Verification items for the finished model (mm, model axes). Face numbers are marked on the shaded views. A direction names the side the tool comes from. Round coordinates to 2 decimals unless told otherwise and drop trailing zeros. Write each loop counter-clockwise with the first axis right and the second up, starting at its lowest first coordinate (ties: lowest second). Pieces come first, ordered by that corner, then holes.
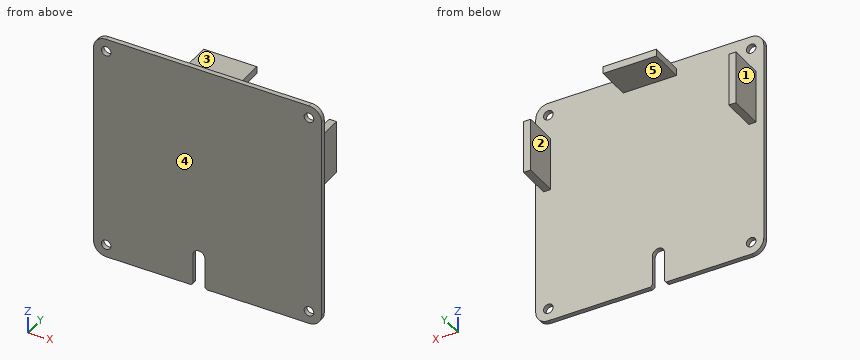
from build123d import *

# Parameters (mm, degrees)
BASE_PLATE_R            = 1.6
PCB_DEPTH               = 1.55
FILLET_1_R              = 1
SKETCH_2_W              = 2.4
SKETCH_2_H              = 17.8
SKETCH_2_W_2            = 17.8
SKETCH_2_H_2            = 2.4
LIDAR_PINS_DEPTH        = 8.5
SKETCH_3_W              = 2.4
SKETCH_3_H              = 17.8
SKETCH_3_W_2            = 17.8
SKETCH_3_H_2            = 2.4
LIDAR_PIN_HEADERS_DEPTH = 3


with BuildPart() as part:
    # Base plate → PCB (new body)
    with BuildSketch(Plane(origin=(0, 0, 0), x_dir=(1, 0, 0), z_dir=(0, 1, 0))):
        with BuildLine():
            ThreePointArc((-38.1, -33.9), (-36.869848481, -36.869848481), (-33.9, -38.1))
            Line((-33.9, -38.1), (33.9, -38.1))
            ThreePointArc((33.9, -38.1), (36.869848481, -36.869848481), (38.1, -33.9))
            Line((38.1, -33.9), (38.1, 33.9))
            ThreePointArc((38.1, 33.9), (36.869848481, 36.869848481), (33.9, 38.1))
            Line((33.9, 38.1), (-0.9, 38.1))
            Line((-0.9, 38.1), (-0.9, 27.4))
            ThreePointArc((-0.9, 27.4), (-2.9, 25.4), (-4.9, 27.4))
            Line((-4.9, 27.4), (-4.9, 38.1))
            Line((-4.9, 38.1), (-33.9, 38.1))
            ThreePointArc((-33.9, 38.1), (-36.869848481, 36.869848481), (-38.1, 33.9))
            Line((-38.1, 33.9), (-38.1, -33.9))
        make_face()
        with Locations(Location((-33.9, -33.9, 0), (0, 0, 90))):
            Circle(BASE_PLATE_R, mode=Mode.SUBTRACT)
        with Locations(Location((33.9, -33.9, 0), (0, 0, 90))):
            Circle(BASE_PLATE_R, mode=Mode.SUBTRACT)
        with Locations(Location((-33.9, 33.9, 0), (0, 0, 90))):
            Circle(BASE_PLATE_R, mode=Mode.SUBTRACT)
        with Locations(Location((33.9, 33.9, 0), (0, 0, 90))):
            Circle(BASE_PLATE_R, mode=Mode.SUBTRACT)
    extrude(amount=PCB_DEPTH)

    # 圆角1
    fillet_1_edges = [part.edges().sort_by_distance(p)[0] for p in [
        (-0.9, 0.775, -38.1),
        (-4.9, 0.775, -38.1),
    ]]
    fillet(fillet_1_edges, radius=FILLET_1_R)

    # 草图2 → Lidar pins (add)
    with BuildSketch(Plane(origin=(0, 1.55, 0), x_dir=(1, 0, 0), z_dir=(0, 1, 0))):
        with Locations((-34.3, -16.5)):
            Rectangle(SKETCH_2_W, SKETCH_2_H)
        with Locations((34.3, -16.5)):
            Rectangle(SKETCH_2_W, SKETCH_2_H)
        with Locations((0, -34.3)):
            Rectangle(SKETCH_2_W_2, SKETCH_2_H_2)
    extrude(amount=LIDAR_PINS_DEPTH)

    # 草图3 → Lidar pin headers (add)
    with BuildSketch(Plane(origin=(0, 10.05, 0), x_dir=(1, 0, 0), z_dir=(0, 1, 0))):
        with Locations((-34.3, -16.5)):
            Rectangle(SKETCH_3_W, SKETCH_3_H)
        with Locations((0, -34.3)):
            Rectangle(SKETCH_3_W_2, SKETCH_3_H_2)
        with Locations((34.3, -16.5)):
            Rectangle(SKETCH_3_W, SKETCH_3_H)
    extrude(amount=LIDAR_PIN_HEADERS_DEPTH)


solid = part.part
Q1. Sectioned sample at D-D (z = 2). Enter the section's corners in (x, y), plus the area to 3 significant figures.
Recorded:
outline: (-38.1, 0) - (38.1, 0) - (38.1, 1.55) - (-38.1, 1.55) - close
area: 118 mm2
Q2. Sectioned sample at C-C (x = 8). Enter the section's corners in (y, z).
Recorded:
outline: (0, -38.1) - (1.55, -38.1) - (1.55, 33.1) - (13.05, 33.1) - (13.05, 35.5) - (1.55, 35.5) - (1.55, 38.1) - (0, 38.1) - close
Q3. Sectioned sample at A-A (y = 8.5). Enter the section's corners in (x, z), plus the area to 3 significant figures.
Recorded:
outline: (-35.5, 7.6) - (-33.1, 7.6) - (-33.1, 25.4) - (-35.5, 25.4) - close; (-8.9, 33.1) - (8.9, 33.1) - (8.9, 35.5) - (-8.9, 35.5) - close; (33.1, 7.6) - (35.5, 7.6) - (35.5, 25.4) - (33.1, 25.4) - close
area: 128 mm2
Q4. Release check for a two-part mould opening along X. For the marked faces 1, 2 and 3 record: released by +X, released by -X, zero draft, split by the parting line, or undercut.
Recorded:
face 1: released by -X
face 2: undercut
face 3: zero draft
Q5. Depth check by flat-ended pin: P1, Ø0.7, axis at x = 33.5, y = 9.5, coming from the +Z side; P2, Ø8, axis at x = 16, z = -22.5, coming from the +Y side; P3, Ø3.5, axis at y = 8, z = 18.5, coming from the -X side. Enter the tip coordinate at first touch or a pass-through.
Recorded:
P1: stops at z = 25.4
P2: stops at y = 1.55
P3: stops at x = -35.5
Q6. Sectioned sample at B-B (z = -29). Enter the section's corners in (x, y).
Recorded:
outline: (-38.1, 0) - (-4.9, 0) - (-4.9, 1.55) - (-38.1, 1.55) - close; (-0.9, 0) - (38.1, 0) - (38.1, 1.55) - (-0.9, 1.55) - close
Q7. Material ranges on line 1 along Z through (x, y) = (33.9, 0.5); line 2 along X through (y, z) = (2.5, 17), recorded low to high.
Recorded:
line 1: z = -38.1 to -35.5, -32.3 to 32.3, 35.5 to 38.1
line 2: x = -35.5 to -33.1, 33.1 to 35.5
Q8. Tool access check on the marked faces 4 and 5. Record the directions out of +Z, -Z, +X, -X, +Y, -Y that give a thin tool (end or side, any length) a straight path to the whole face; none if there is none.
Recorded:
face 4: +Z, -Z, +X, -X, -Y
face 5: -Z, +X, -X, +Y
